Build history of the part. All positions in model axes, mm. Face numbers are marked on the shaded views. A direction names the side the tool comes from. Coordinates: 2 decimals unless noted, no trailing zeros. Loops run counter-clockwise (first coordinate to the right, second up) from the corner with the lowest first, then second, coordinate; pieces in that order, holes last.
(1) Slice it at B-B (y = 26). Give the cut face in (x, z).
(2) Slice it at D-D (z = -10.75). Give the cut face in (x, y), and give its area (3 significant figures).
(3) Wall check: L1, parallel to X at y = 13, z = -5.25; L2, parallel to Y at x = 0, z = -0.8. Give the ranges that are in metal, low to high.
(4) Two-plate mould, pull along X, no slides. Class the marked faces 1, 2 and 3: pulls with the +X half, pulls with the -X half, needs draft (parallel to the pull), parting line crosses it, or undercut.
(5) Flat gauge pins, fed straight in: P1, Ø3, axis at x = -1, z = -5, coming from the +Y side; P2, Ø2, axis at x = 0, y = -37, coming from the +Z side; P3, Ø5.5, axis at y = 0, z = -6, coming from the +X side. Where does each tip first touch, or does it go through?
(6) Tool access for the marked faces 4 and 5: list every direction of +Z, -Z, +X, -X, +Y, -Y with a clear straight run to the whole face (end or side of a thin tool).
from build123d import *

# Parameters (mm, degrees)
F0_W      = 85
F0_H      = 85
F0_R      = 2
F1_DEPTH  = 20
F2_DEPTH  = 15
F3_R      = 5
F4_R      = 3
F5_R      = 1
F6_R      = 3.1
F7_DEPTH  = 3.1
F8_R      = 3.1
F9_DEPTH  = 3.1
F10_R     = 3.1
F11_DEPTH = 3.1
F12_R     = 3.1
F13_DEPTH = 3.1
F14_DEPTH = 1
F15_ANGLE = 180


# Not quite as in the source:
# - a feature names something its author has since deleted; it is built from what else it names


with BuildPart() as f1:
    # F0 (on Top) → F1 (new body)
    with BuildSketch(Plane.XY):
        Rectangle(F0_W, F0_H)
        with Locations((0, -37.75)):
            Circle(F0_R, mode=Mode.SUBTRACT)
        with BuildLine():
            ThreePointArc((-33, 30), (-32.1213203436, 32.1213203436), (-30, 33))
            Line((-30, 33), (30, 33))
            ThreePointArc((30, 33), (32.1213203436, 32.1213203436), (33, 30))
            Line((33, 30), (33, -30))
            ThreePointArc((33, -30), (32.1213203436, -32.1213203436), (30, -33))
            Line((30, -33), (-30, -33))
            ThreePointArc((-30, -33), (-32.1213203436, -32.1213203436), (-33, -30))
            Line((-33, -30), (-33, 30))
        make_face(mode=Mode.SUBTRACT)
        with BuildLine():
            Line((30, 33), (-30, 33))
            ThreePointArc((-30, 33), (-32.1213203436, 32.1213203436), (-33, 30))
            Line((-33, 30), (-33, -30))
            ThreePointArc((-33, -30), (-32.1213203436, -32.1213203436), (-30, -33))
            Line((-30, -33), (30, -33))
            ThreePointArc((30, -33), (32.1213203436, -32.1213203436), (33, -30))
            Line((33, -30), (33, 30))
            ThreePointArc((33, 30), (32.1213203436, 32.1213203436), (30, 33))
        make_face()
        with Locations((0, -37.75)):
            Circle(F0_R)
    extrude(amount=F1_DEPTH)

    # F0 (on Top) → F2 (cut)
    with BuildSketch(Plane.XY):
        with BuildLine():
            Line((30, 33), (-30, 33))
            ThreePointArc((-30, 33), (-32.1213203436, 32.1213203436), (-33, 30))
            Line((-33, 30), (-33, -30))
            ThreePointArc((-33, -30), (-32.1213203436, -32.1213203436), (-30, -33))
            Line((-30, -33), (30, -33))
            ThreePointArc((30, -33), (32.1213203436, -32.1213203436), (33, -30))
            Line((33, -30), (33, 30))
            ThreePointArc((33, 30), (32.1213203436, 32.1213203436), (30, 33))
        make_face()
    extrude(amount=F2_DEPTH, mode=Mode.SUBTRACT)

    # F3
    f3_edges = [f1.edges().sort_by_distance(p)[0] for p in [
        (0, 42.5, 20),
        (-42.5, 0, 20),
        (0, -42.5, 20),
        (42.5, 0, 20),
        (42.5, 42.5, 10),
        (-42.5, 42.5, 10),
        (-42.5, -42.5, 10),
        (42.5, -42.5, 10),
    ]]
    fillet(f3_edges, radius=F3_R)

    # F4
    f4_edges = [f1.edges().sort_by_distance(p)[0] for p in [
        (0, 33, 15),
        (-32.12132, 32.12132, 15),
        (-33, 0, 15),
        (-32.12132, -32.12132, 15),
        (0, -33, 15),
        (32.12132, -32.12132, 15),
        (33, 0, 15),
        (32.12132, 32.12132, 15),
    ]]
    fillet(f4_edges, radius=F4_R)

    # F5
    f5_edges = [f1.edges().sort_by_distance(p)[0] for p in [
        (0, 42.5, 0),
        (41.035534, 41.035534, 0),
        (-41.035534, 41.035534, 0),
        (42.5, 0, 0),
        (-42.5, 0, 0),
        (41.035534, -41.035534, 0),
        (-41.035534, -41.035534, 0),
        (0, -42.5, 0),
        (0, 33, 0),
        (-32.12132, 32.12132, 0),
        (-33, 0, 0),
        (-32.12132, -32.12132, 0),
        (0, -33, 0),
        (32.12132, -32.12132, 0),
        (33, 0, 0),
        (32.12132, 32.12132, 0),
    ]]
    fillet(f5_edges, radius=F5_R)

    # F6 (on face) → F7 (cut)
    with BuildSketch(Plane.XZ.offset(42.5)):
        with Locations((0, 6)):
            Circle(F6_R)
    extrude(amount=-F7_DEPTH, mode=Mode.SUBTRACT)

    # F8 (on face) → F9 (cut)
    with BuildSketch(Plane(origin=(0, 42.5, 0), x_dir=(-1, 0, 0), z_dir=(0, 1, 0))):
        with Locations((0, 6)):
            Circle(F8_R)
    extrude(amount=-F9_DEPTH, mode=Mode.SUBTRACT)

    # F10 (on face) → F11 (cut)
    with BuildSketch(Plane(origin=(-42.5, 0, 0), x_dir=(0, -1, 0), z_dir=(-1, 0, 0))):
        with Locations((0, 6)):
            Circle(F10_R)
    extrude(amount=-F11_DEPTH, mode=Mode.SUBTRACT)

    # F12 (on face) → F13 (cut)
    with BuildSketch(Plane.YZ.offset(42.5)):
        with Locations((0, 6)):
            Circle(F12_R)
    extrude(amount=-F13_DEPTH, mode=Mode.SUBTRACT)

    # F0 (on Top) → F14 (cut)
    with BuildSketch(Plane.XY):
        with Locations((0, -37.75)):
            Circle(F0_R)
    extrude(amount=F14_DEPTH, mode=Mode.SUBTRACT)


with BuildPart() as f1_1:
    # F15: moved
    add(f1.part.rotate(Axis((0, 0, 0), (0, 1, 0)), F15_ANGLE))


solid = f1_1.part
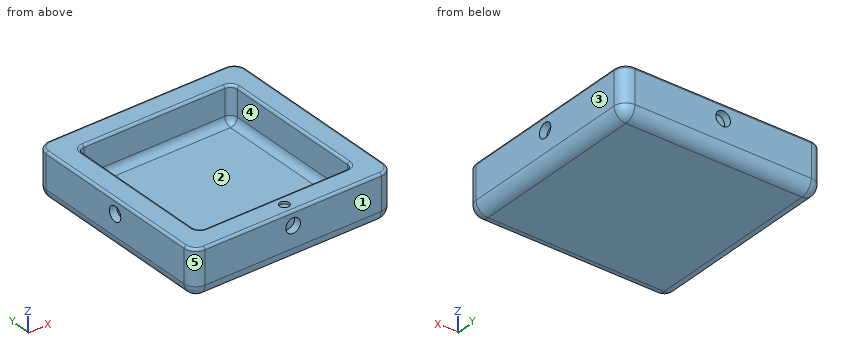
Response values:
1. outline: (-42.5, -15) arc R5 ccw to (-37.5, -20) - (37.5, -20) arc R5 ccw to (42.5, -15) - (42.5, -1) arc R1 ccw to (41.5, 0) - (34, 0) arc R1 ccw to (33, -1) - (33, -12) arc R3 cw to (30, -15) - (-30, -15) arc R3 cw to (-33, -12) - (-33, -1) arc R1 ccw to (-34, 0) - (-41.5, 0) arc R1 ccw to (-42.5, -1) - close
2. outline: (-42.5, -37.5) arc R5 ccw to (-37.5, -42.5) - (37.5, -42.5) arc R5 ccw to (42.5, -37.5) - (42.5, 37.5) arc R5 ccw to (37.5, 42.5) - (-37.5, 42.5) arc R5 ccw to (-42.5, 37.5) - close; hole (-33, -30) arc R3 ccw to (-30, -33) - (30, -33) arc R3 ccw to (33, -30) - (33, 30) arc R3 ccw to (30, 33) - (-30, 33) arc R3 ccw to (-33, 30) - close
2. area: 2,860 mm2
3. L1: x = -42.5 to -33, 33 to 42.5
3. L2: y = -42.48 to -39.75, -35.75 to -33.02, 33.02 to 42.48
4. face 1: needs draft
4. face 2: undercut
4. face 3: pulls with the +X half
5. P1: stops at y = 39.4
5. P2: stops at z = -1
5. P3: stops at x = 39.4
6. face 4: +Z
6. face 5: +Z, -Z, -X, -Y
